Build history of the part. All positions in model axes, mm. A direction names the side the tool comes from. Give positions to 0.01 mm unless a question says otherwise; leave off trailing zeros. Order: outer loops, then holes, each group sorted by start corner. A loop starts at its lowest first (then second) coordinate and runs counter-clockwise, first axis right, second up. Notation, with made-up numbers: (82.5, -19.75) - (114.5, -19.75) arc R10 ccw to (114.5, -6.75) - close; hole circle Ø2 at (-10.5, -38). An arc over 180 degrees is marked (long way). One line per item, written item: value.
```python
from build123d import *

# Parameters (mm, degrees)
BOSS_EXTRUDE1_DEPTH = 10
SKETCH2_W           = 168.929390661
SKETCH2_H           = 12
CUT_EXTRUDE1_DEPTH  = 6
SKETCH3_W           = 79.959911579
SKETCH3_H           = 12
CUT_EXTRUDE2_DEPTH  = 6


with BuildPart() as part:
    # Sketch1 → Boss-Extrude1 (new body)
    with BuildSketch(Plane.XY):
        with BuildLine():
            Line((85.170110947, 22.083871035), (267.939703111, 22.083871035))
            ThreePointArc((267.939703111, 22.083871035), (282.081838735, 16.226006659), (287.939703111, 2.083871035))
            Line((287.939703111, 2.083871035), (287.939703111, -2.083871035))
            ThreePointArc((287.939703111, -2.083871035), (282.081838735, -16.226006659), (267.939703111, -22.083871035))
            Line((267.939703111, -22.083871035), (85.170110947, -22.083871035))
            ThreePointArc((85.170110947, -22.083871035), (74.615378512, -25.095709768), (67.239561274, -33.224108712))
            ThreePointArc((67.239561274, -33.224108712), (-75, 0), (67.239561274, 33.224108712))
            ThreePointArc((67.239561274, 33.224108712), (74.615378512, 25.095709768), (85.170110947, 22.083871035))
        make_face()
    extrude(amount=BOSS_EXTRUDE1_DEPTH)

    # Sketch2 → Cut-Extrude1 (cut)
    with BuildSketch(Plane.XY.offset(10)):
        with Locations((194.3131347, -1.883371564)):
            Rectangle(SKETCH2_W, SKETCH2_H)
    extrude(amount=-CUT_EXTRUDE1_DEPTH, mode=Mode.SUBTRACT)

    # Sketch3 → Cut-Extrude2 (cut)
    with BuildSketch(Plane.XY.offset(10)):
        with Locations((318.757785819, -1.883371564)):
            Rectangle(SKETCH3_W, SKETCH3_H)
    extrude(amount=-CUT_EXTRUDE2_DEPTH, mode=Mode.SUBTRACT)


solid = part.part
```
(1) Pin check, flat tips, straight feed: P1, Ø1.8, axis at y = -1.5, z = 7, coming from the +X side; P2, Ø5, axis at y = -22, z = 4.5, coming from the -X side; P3, Ø3, axis at x = 155.5, z = 8, coming from the -Y side. Stop position of each tip, or through.
Completed:
P1: x = 109.85
P2: x = -72.42
P3: y = -22.08
(2) Slice it at B-B, the plane x = 236. Give the cut face in (y, z).
Completed:
outline: (-22.08, 0) - (22.08, 0) - (22.08, 10) - (4.12, 10) - (4.12, 4) - (-7.88, 4) - (-7.88, 10) - (-22.08, 10) - close
(3) Drill centre lines: line 1 (Y direction, x = 157, z = 8); line 2 (Y direction, x = 92, z = 9.5); line 3 (Y direction, x = -1, z = 6.75). Where is each one in solid material? Low to high.
Completed:
line 1: -22.08 to -7.88, 4.12 to 22.08
line 2: -22.08 to 22.08
line 3: -74.99 to 74.99
(4) Pull direction Y, two halves, no side cores. Call faces 4 (the face through (69, 1, 0)), 5 (the face through (178, -22.084, 5)), 6 (the face through (198, -2, 4)): +Y half, -Y half, draft (parallel to the pull), parting line (faces both ways), or undercut.
Completed:
face 4: draft
face 5: -Y half
face 6: undercut
(5) Slice it at C-C, the plane y = 59. Give the cut face in (x, z), and give its area (3 significant figures).
Completed:
outline: (-46.3, 0) - (46.3, 0) - (46.3, 10) - (-46.3, 10) - close
area: 926 mm²
(6) 3-axis set-ups, long thin cutter, end or side, ignore diameter. For faces 1 (the face through (109.848, -2, 7)), 2 (the face through (175, 22.084, 5)), 3 (the face through (279.59, -18.34, 4.93)): which of +Z, -Z, +X, -X, +Y, -Y reach the whole face in a straight line?
Completed:
face 1: +Z, +X
face 2: +Z, -Z, +X, +Y
face 3: +Z, -Z, +X, -Y
(7) Slice it at A-A, the plane z = 2.25. Give the cut face in (x, y).
Completed:
outline: (67.24, -33.22) arc R20 cw to (85.17, -22.08) - (267.94, -22.08) arc R20 ccw to (287.94, -2.08) - (287.94, 2.08) arc R20 ccw to (267.94, 22.08) - (85.17, 22.08) arc R20 cw to (67.24, 33.22) arc R75 ccw (long way) to start
(8) Slice it at D-D, the plane x = 72. Give the cut face in (y, z).
Completed:
outline: (-27.03, 0) - (27.03, 0) - (27.03, 10) - (-27.03, 10) - close
